```python
from build123d import *

# Parameters (mm, degrees)
F0_R     = 63.5
F0_R_2   = 12.7
F0_R_3   = 6.35
F1_DEPTH = 25.4
F2_SIZE  = 0.0508


with BuildPart() as f1:
    # F0 (on Front) → F1 (new body)
    with BuildSketch(Plane.XZ):
        Circle(F0_R)
        Circle(F0_R_2, mode=Mode.SUBTRACT)
        with Locations((0, 51.805038)):
            Circle(F0_R_3, mode=Mode.SUBTRACT)
    extrude(amount=F1_DEPTH)

    # F2
    f2_edges = [f1.edges().sort_by_distance(p)[0] for p in [
        (12.7, -12.7, 0),
        (-12.7, 0, 0),
        (-12.7, -25.4, 0),
    ]]
    chamfer(f2_edges, length=F2_SIZE)


solid = f1.part
```
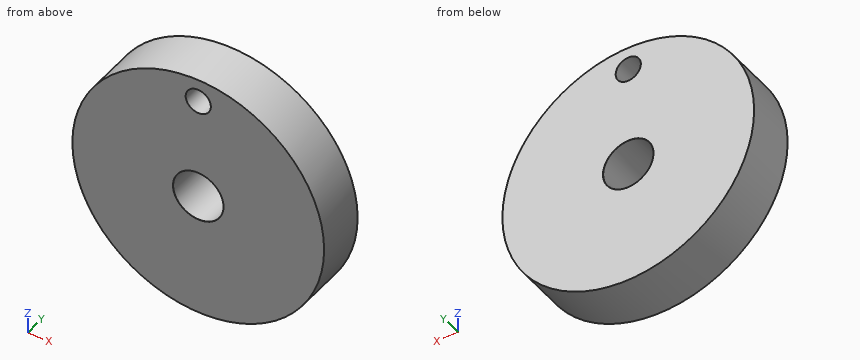
The model under review builds one solid part; all positions refer to its coordinate system, in mm. Round coordinates to 2 decimals unless told otherwise and drop trailing zeros. Loops run counter-clockwise (first coordinate to the right, second up) from the corner with the lowest first, then second, coordinate; pieces in that order, holes last. Notation, with made-up numbers: (49.25, 78.25) -> (98.25, 78.25) arc R15 cw to (98.25, 96.25) -> close; hole circle Ø8 at (61.25, 64.25). An arc over 180 degrees is marked (long way). Answer in a Markdown table with one row per item.
1) Consider section B-B, the plane x = 0. Write out the cut boundary in (y, z).
Taken from the geometry:
| item | result |
|---|---|
| outline | (-25.4, -63.5) -> (0, -63.5) -> (0, -12.75) -> (-0.05, -12.7) -> (-25.35, -12.7) -> (-25.4, -12.75) -> close; (-25.4, 12.75) -> (-25.35, 12.7) -> (-0.05, 12.7) -> (0, 12.75) -> (0, 45.46) -> (-25.4, 45.46) -> close; (-25.4, 58.16) -> (0, 58.16) -> (0, 63.5) -> (-25.4, 63.5) -> close |
2) Consider section C-C, the plane y = -22. Write out the cut boundary in (x, z), plus the area to 3 significant figures.
Taken from the geometry:
| item | result |
|---|---|
| outline | circle Ø127 at (0, 0); hole circle Ø25.4 at (0, 0); hole circle Ø12.7 at (0, 51.81) |
| area | 12,000 mm² |
3) Consider section D-D, the plane z = 17. Write out the cut boundary in (x, y).
Taken from the geometry:
| item | result |
|---|---|
| outline | (-61.18, -25.4) -> (61.18, -25.4) -> (61.18, 0) -> (-61.18, 0) -> close |
4) Consider section A-A, the plane z = 0. Write out the cut boundary in (x, y), plus the area to 3 significant figures.
Taken from the geometry:
| item | result |
|---|---|
| outline | (-63.5, -25.4) -> (-12.75, -25.4) -> (-12.7, -25.35) -> (-12.7, -0.05) -> (-12.75, 0) -> (-63.5, 0) -> close; (12.7, -25.35) -> (12.75, -25.4) -> (63.5, -25.4) -> (63.5, 0) -> (12.75, 0) -> (12.7, -0.05) -> close |
| area | 2,580 mm² |
5) For pin 1 Ø1 at (x, y) = (3, -17) entering from -Z; pin 2 Ø1 at (x, y) = (-34, -20) entering from +Z; pin 3 Ø6 at (x, y) = (36.5, -6) entering from -Z; pin 4 Ø11.5 at (x, z) = (0, 51.81) entering from -Y, all flat-tipped, find the tip position at first contact; note any pin that passes through.
Taken from the geometry:
| item | result |
|---|---|
| pin 1 | stops at z = -63.45 |
| pin 2 | stops at z = 53.94 |
| pin 3 | stops at z = -53.94 |
| pin 4 | passes through |
6) Wall thickness on line 1 along Z through (x, y) = (0, -16.25); line 2 along Z through (x, y) = (0.5, -16.25); line 3 along Z through (x, y) = (-9.5, -17.25): over which ranges is each line inside the solid? List them lowest first.
Taken from the geometry:
| item | result |
|---|---|
| line 1 | z = -63.5 to -12.7, 12.7 to 45.46, 58.16 to 63.5 |
| line 2 | z = -63.5 to -12.69, 12.69 to 45.47, 58.14 to 63.5 |
| line 3 | z = -62.79 to -8.43, 8.43 to 62.79 |
